For this review, take the finished solid that the model builds, in its own axes (mm). A direction names the side the tool comes from. Give positions to 0.01 mm unless a question says otherwise; leave off trailing zeros. Order: outer loops, then holes, each group sorted by start corner. A loop starts at its lowest first (then second) coordinate and runs counter-clockwise, first axis right, second up.
from build123d import *

# Parameters (mm, degrees)
SKETCH062_R     = 1.1
SKETCH062_R_2   = 1
PAD027_DEPTH    = 2
SKETCH063_R     = 2.4
SKETCH063_R_2   = 1
PAD028_DEPTH    = 17
SKETCH064_R     = 2.4
SKETCH064_R_2   = 1
PAD029_DEPTH    = 9
SKETCH065_R     = 2.1
SKETCH065_R_2   = 1.1
PAD030_DEPTH    = 20
POCKET029_DEPTH = 15
POCKET030_DEPTH = 59.501
SKETCH068_W     = 5
SKETCH068_H     = 3
SKETCH068_H_2   = 5
POCKET031_DEPTH = 5
SKETCH069_R     = 3.1
POCKET032_DEPTH = 8
POCKET033_DEPTH = 6
POCKET034_DEPTH = 7
CHAMFER004_SIZE = 0.8


with BuildPart() as part:
    # Sketch062 → Pad027 (new body)
    with BuildSketch(Plane(origin=(51, -95, 6), x_dir=(1, 0, 0), z_dir=(0, 0, -1))):
        with BuildLine():
            Line((0, 0), (-60, 0))
            Line((-60, 0), (-70.068466, 16.112914))
            ThreePointArc((-68, 20), (-70.213604, 18.684045), (-70.068466, 16.112914))
            Line((0, 20), (-68, 20))
            Line((0, 0), (0, 20))
        make_face()
        with Locations((-2.5, 2.5)):
            Circle(SKETCH062_R, mode=Mode.SUBTRACT)
        with Locations((-2.5, 17.5)):
            Circle(SKETCH062_R, mode=Mode.SUBTRACT)
        with Locations((-14.5, 17.5)):
            Circle(SKETCH062_R, mode=Mode.SUBTRACT)
        with Locations((-14.5, 2.5)):
            Circle(SKETCH062_R, mode=Mode.SUBTRACT)
        with Locations((-45, 2.5)):
            Circle(SKETCH062_R, mode=Mode.SUBTRACT)
        with Locations((-57, 2.5)):
            Circle(SKETCH062_R, mode=Mode.SUBTRACT)
        with Locations((-57, 17.5)):
            Circle(SKETCH062_R, mode=Mode.SUBTRACT)
        with Locations((-68.022489, 17.518069)):
            Circle(SKETCH062_R_2, mode=Mode.SUBTRACT)
        with Locations((-37, 17)):
            Circle(SKETCH062_R_2, mode=Mode.SUBTRACT)
    extrude(amount=PAD027_DEPTH)

    # Sketch063 → Pad028 (new body)
    with BuildSketch(Plane(origin=(51, -95, 4), x_dir=(1, 0, 0), z_dir=(0, 0, -1))):
        with Locations((-68.022489, 17.518069)):
            Circle(SKETCH063_R)
        with Locations((-68.022489, 17.518069)):
            Circle(SKETCH063_R_2, mode=Mode.SUBTRACT)
    extrude(amount=PAD028_DEPTH)

    # Sketch064 → Pad029 (new body)
    with BuildSketch(Plane(origin=(51, -95, 4), x_dir=(1, 0, 0), z_dir=(0, 0, -1))):
        with Locations((-37, 17)):
            Circle(SKETCH064_R)
        with Locations((-37, 17)):
            Circle(SKETCH064_R_2, mode=Mode.SUBTRACT)
    extrude(amount=PAD029_DEPTH)

    # Sketch065 → Pad030 (new body)
    with BuildSketch(Plane(origin=(51, -95, 4), x_dir=(1, 0, 0), z_dir=(0, 0, -1))):
        Polygon((0, 0), (-24.5, 0), (-24.5, 30), (-14.5, 30), (-14.5, 10), (0, 10), align=None)
        with Locations((-19.5, 25)):
            Circle(SKETCH065_R, mode=Mode.SUBTRACT)
        with Locations((-14.5, 2.5)):
            Circle(SKETCH065_R_2, mode=Mode.SUBTRACT)
        with Locations((-2.5, 2.5)):
            Circle(SKETCH065_R_2, mode=Mode.SUBTRACT)
        Polygon((-59.5, 0), (-42.5, 0), (-42.5, 10), (-49.5, 10), (-49.5, 30), (-59.5, 30), align=None)
        with Locations((-54.5, 25)):
            Circle(SKETCH065_R, mode=Mode.SUBTRACT)
        with Locations((-57, 2.5)):
            Circle(SKETCH065_R_2, mode=Mode.SUBTRACT)
        with Locations((-45, 2.5)):
            Circle(SKETCH065_R_2, mode=Mode.SUBTRACT)
        with Locations((-57, 17.5)):
            Circle(SKETCH065_R_2, mode=Mode.SUBTRACT)
    extrude(amount=PAD030_DEPTH)

    # Sketch066 → Pocket029 (cut)
    with BuildSketch(Plane(origin=(51, -95, 4), x_dir=(1, 0, 0), z_dir=(0, 0, 1))):
        Polygon((-51.035898, -27), (-51.035898, -23), (-54.5, -21), (-57.964102, -23), (-57.964102, -27), (-54.5, -29), align=None)
        Polygon((-16.035898, -27), (-16.035898, -23), (-19.5, -21), (-22.964102, -23), (-22.964102, -27), (-19.5, -29), align=None)
    extrude(amount=-POCKET029_DEPTH, mode=Mode.SUBTRACT)

    # Sketch067 → Pocket030 (cut, through all)
    with BuildSketch(Plane(origin=(-8.5, -95, 6), x_dir=(0, 1, 0), z_dir=(-1, 0, 0))):
        Polygon((-22.58819, 11.659258), (-30, 17), (-30, 2), (-20, 2), align=None)
        Polygon((0, 22), (0, 12), (-10, 12), (-15, 22), align=None)
    extrude(amount=-POCKET030_DEPTH, mode=Mode.SUBTRACT)

    # Sketch068 → Pocket031 (cut)
    with BuildSketch(Plane(origin=(-8.5, -95, 6), x_dir=(0, 1, 0), z_dir=(-1, 0, 0))):
        with Locations((-17.5, 20.5)):
            Rectangle(SKETCH068_W, SKETCH068_H)
        with Locations((-17.5, 11.5)):
            Rectangle(SKETCH068_W, SKETCH068_H_2)
    extrude(amount=-POCKET031_DEPTH, mode=Mode.SUBTRACT)

    # Sketch069 → Pocket032 (cut)
    with BuildSketch(Plane(origin=(51, -95, 6), x_dir=(1, 0, 0), z_dir=(0, 1, 0))):
        with Locations((-8.5, 6)):
            Circle(SKETCH069_R)
        with Locations((-51, 6)):
            Circle(SKETCH069_R)
    extrude(amount=-POCKET032_DEPTH, mode=Mode.SUBTRACT)

    # Sketch070 → Pocket033 (cut, symmetric)
    with BuildSketch(Plane(origin=(51, -95, -3), x_dir=(1, 0, 0), z_dir=(0, 0, -1))):
        Polygon((-55.008142, 16.35), (-55.008142, 18.65), (-57, 19.8), (-58.991858, 18.65), (-58.991858, 16.35), (-57, 15.2), align=None)
    extrude(amount=POCKET033_DEPTH, both=True, mode=Mode.SUBTRACT)

    # Sketch071 → Pocket034 (cut)
    with BuildSketch(Plane(origin=(26.5, -95, 6), x_dir=(0, 1, 0), z_dir=(-1, 0, 0))):
        Polygon((-10, 12), (0, 2), (0, 12), align=None)
    extrude(amount=-POCKET034_DEPTH, mode=Mode.SUBTRACT)

    # Chamfer004
    chamfer004_edges = [part.edges().sort_by_distance(p)[0] for p in [
        (17, -115, 6),
        (29.4, -120, -11),
        (-5.6, -120, -11),
        (-7.1, -112.5, -9),
    ]]
    chamfer(chamfer004_edges, length=CHAMFER004_SIZE)


solid = part.part
1) We need section C-C on z = -1.5. Count the separate pieces of the cut face and the enclosed holes in it, then the cut area to 3 significant figures.
Answer sheet:
separate pieces: 4
enclosed holes: 7
area: 519 mm2
2) To check wall thickness, follow line 1 (Y direction, x = -6, z = 3.95); line 2 (X direction, y = -108.75, z = 0.5); line 3 (Z direction, x = 42.5, y = -101). State the ranges of each line that lie inside material, in increasing order.
Answer sheet:
line 1: y = -115.01 to -113.6, -111.4 to -98.6, -96.4 to -95
line 2: x = -8.5 to 1.5, 26.5 to 36.5
line 3: z = -6 to -3.1, 3.1 to 6
3) Draft analysis for pull direction Z (two halves, no side actions). For faces 1 (the face through (26.5, -110, -6)), 2 (the face through (29, -122, -11)), 3 (the face through (-3.5, -113, -6)), state which applies: +Z half, -Z half, draft (parallel to the pull), parting line (faces both ways), or undercut.
Answer sheet:
face 1: draft
face 2: +Z half
face 3: undercut
4) Tool access review of faces 4 (the face through (-5.641, -122.764, -10.144)), 5 (the face through (-4.99, -114.217, -0.042)), 6 (the face through (42, -100, -6)): name each direction out of +Z, -Z, +X, -X, +Y, -Y from which nothing blocks a thin tool from reaching the whole face with its end or side.
Answer sheet:
face 4: +Z
face 5: none
face 6: -Z, +X, -X, +Y
5) We need section D-D on y = -108.5. Give the boundary of the cut face in (x, z).
Answer sheet:
outline: (-17.44, 4) - (-8.5, 4) - (-8.5, -13) - (1.5, -13) - (1.5, 4) - (26.5, 4) - (26.5, -13) - (36.5, -13) - (36.5, 4) - (51, 4) - (51, 6) - (-16.49, 6) - (-17.44, 5.2) - close
6) We need section A-A on x = 6. Give the boundary of the cut face in (y, z), then the cut area to 3 significant figures.
Answer sheet:
outline: (-115, 4) - (-105, 4) - (-105, -6) - (-98.6, -6) - (-98.6, 6) - (-114.2, 6) - (-115, 5.2) - close; (-96.4, -6) - (-95, -6) - (-95, 6) - (-96.4, 6) - close
area: 113 mm2
7) We need section B-B on x = 48.5. Give the boundary of the cut face in (y, z), then the cut area to 3 significant figures.
Answer sheet:
outline: (-115, 4) - (-113.6, 4) - (-113.6, 6) - (-114.2, 6) - (-115, 5.2) - close; (-111.4, 4) - (-105, 4) - (-105, -6) - (-98.6, -6) - (-98.6, 6) - (-111.4, 6) - close; (-96.4, -6) - (-95, -6) - (-95, 6) - (-96.4, 6) - close
area: 109 mm2
8) Clearance check with flat-ended pins moving along their axes: pin 1 (3 mm diameter, centred on y = -100.5, z = -2.5, fed in from -X); pin 2 (3 mm diameter, centred on y = -121, z = -9.5, fed in from +X); pin 3 (5 mm diameter, centred on x = -9.5, z = 0.5, fed in from -Y). State where each tip first meets the part, or that it passes through.
Answer sheet:
pin 1: stops at x = -8.5
pin 2: stops at x = 36.5
pin 3: stops at y = -116.55
